Verification items for the finished model (mm, model axes). Face numbers are marked on the shaded views. A direction names the side the tool comes from. Round coordinates to 2 decimals unless told otherwise and drop trailing zeros. Write each loop counter-clockwise with the first axis right and the second up, starting at its lowest first coordinate (ties: lowest second). Pieces come first, ordered by that corner, then holes. Notation, with made-up numbers: M 11,44.25 L 59,44.25 A34 ccw 59,77.25 Z; hole C 81,57 d2. An arc over 180 degrees is marked long. One line per item, written item: value. Start each with the question number.
Item 1: Tool access check on the marked faces 4, 5 and 6. Record the directions out of +Z, -Z, +X, -X, +Y, -Y that give a thin tool (end or side, any length) a straight path to the whole face; none if there is none.
Item 2: Gauge pin test, flat ends, axial feed: pin 1 (5.5 mm diameter, centred on y = 19.5, z = 13, fed in from +X); pin 2 (5.5 mm diameter, centred on y = 19.5, z = 14.5, fed in from -X); pin 3 (2.5 mm diameter, centred on x = 0, z = 1, fed in from -Y). Record the tip position at first contact, or that the pin passes through.
Item 3: Section check D-D, the plane y = 12.8. State how many separate pieces and enclosed holes the cut face has, then the cut area to 3 significant figures.
Item 4: Section check A-A, the plane y = 16.75. Record the cut outline in (x, z), then the cut area to 3 significant figures.
Item 5: Section check C-C, the plane z = -13.5. Record the cut outline in (x, y), then the cut area to 3 significant figures.
Item 6: Thickness scan on probe 1 along Y at (x, z) = (-18.7, 13.5); probe 2 along X at (y, z) = (15.5, 12); probe 3 along X at (y, z) = (3.55, 0). Record the ranges inside material, lowest first. Write a range as from..to.
Item 7: Draft check along X on the marked faces 1, 2 and 3. Enter one of: +X half, -X half, draft (parallel to the pull), parting line (faces both ways), or undercut.
Item 8: Section check B-B, the plane x = 0. Record the cut outline in (y, z), then the cut area to 3 significant figures.
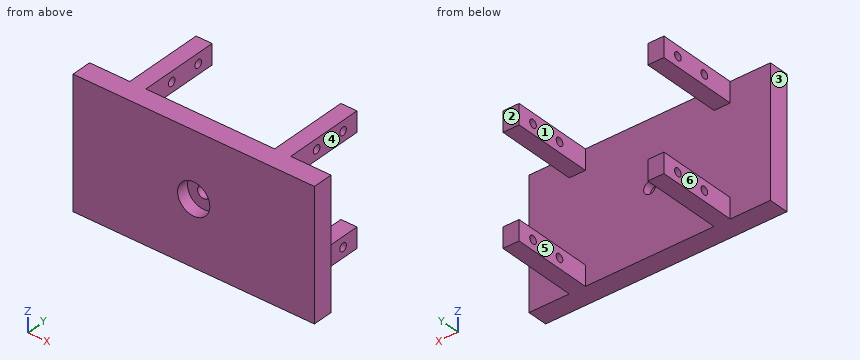
from build123d import *

# Parameters (mm, degrees)
SKETCH1_W           = 60
SKETCH1_H           = 32
SKETCH1_R           = 1.5
BOSS_EXTRUDE1_DEPTH = 5
SKETCH2_R           = 4
CUT_EXTRUDE1_DEPTH  = 3
SKETCH3_W           = 4
SKETCH3_H           = 32
BOSS_EXTRUDE2_DEPTH = 20
SKETCH4_R           = 1
SKETCH4_W           = 22
SKETCH4_H           = 20
CUT_EXTRUDE2_DEPTH  = 59.14636704


with BuildPart() as part:
    # Sketch1 → Boss-Extrude1 (new body)
    with BuildSketch(Plane(origin=(0, 0, 0), x_dir=(1, 0, 0), z_dir=(0, 1, 0))):
        Rectangle(SKETCH1_W, SKETCH1_H)
        with Locations(Location((0, 0, 0), (0, 0, 270))):
            Circle(SKETCH1_R, mode=Mode.SUBTRACT)
    extrude(amount=BOSS_EXTRUDE1_DEPTH)

    # Sketch2 → Cut-Extrude1 (cut)
    with BuildSketch(Plane.XZ):
        with Locations(Location((0, 0, 0), (0, 0, 270))):
            Circle(SKETCH2_R)
    extrude(amount=-CUT_EXTRUDE1_DEPTH, mode=Mode.SUBTRACT)

    # Sketch3 → Boss-Extrude2 (add)
    with BuildSketch(Plane(origin=(0, 5, 0), x_dir=(1, 0, 0), z_dir=(0, 1, 0))):
        with Locations((-18, 0)):
            Rectangle(SKETCH3_W, SKETCH3_H)
        with Locations((18, 0)):
            Rectangle(SKETCH3_W, SKETCH3_H)
    extrude(amount=BOSS_EXTRUDE2_DEPTH)

    # Sketch4 → Cut-Extrude2 (cut, through all)
    with BuildSketch(Plane.ZY.offset(20)):
        with Locations((-13.5, 20.8)):
            Circle(SKETCH4_R)
        with Locations((-13.5, 12.8)):
            Circle(SKETCH4_R)
        with Locations((13.5, 20.8)):
            Circle(SKETCH4_R)
        with Locations((13.5, 12.8)):
            Circle(SKETCH4_R)
        with Locations((0, 15)):
            Rectangle(SKETCH4_W, SKETCH4_H)
    extrude(amount=-CUT_EXTRUDE2_DEPTH, mode=Mode.SUBTRACT)


solid = part.part
Response values:
1. face 4: +Z, -Z, +X, +Y
1. face 5: +Z, -Z, +Y
1. face 6: +Z, -Z, -X, +Y
2. pin 1: stops at x = 20
2. pin 2: stops at x = -20
2. pin 3: stops at y = 3
3. separate pieces: 8
3. enclosed holes: 0
3. area: 48.0 mm2
4. outline: M -20,-16 L -16,-16 L -16,-11 L -20,-11 Z; M -20,11 L -16,11 L -16,16 L -20,16 Z; M 16,-16 L 20,-16 L 20,-11 L 16,-11 Z; M 16,11 L 20,11 L 20,16 L 16,16 Z
4. area: 80.0 mm2
5. outline: M -30,0 L 30,0 L 30,5 L 20,5 L 20,11.8 L 16,11.8 L 16,5 L -16,5 L -16,11.8 L -20,11.8 L -20,5 L -30,5 Z; M -20,13.8 L -16,13.8 L -16,19.8 L -20,19.8 Z; M -20,21.8 L -16,21.8 L -16,25 L -20,25 Z; M 16,13.8 L 20,13.8 L 20,19.8 L 16,19.8 Z; M 16,21.8 L 20,21.8 L 20,25 L 16,25 Z
5. area: 428 mm2
6. probe 1: y = 0..11.8, 13.8..19.8, 21.8..25
6. probe 2: x = -20..-16, 16..20
6. probe 3: x = -30..-1.5, 1.5..30
7. face 1: undercut
7. face 2: draft
7. face 3: -X half
8. outline: M 0,-16 L 5,-16 L 5,-1.5 L 3,-1.5 L 3,-4 L 0,-4 Z; M 0,4 L 3,4 L 3,1.5 L 5,1.5 L 5,16 L 0,16 Z
8. area: 130 mm2
